Verification items for this drawing (mm, ordinates from the low corner). Round coordinates to 2 decimals unless told otherwise and drop trailing zeros. Loops run counter-clockwise (first coordinate to the right, second up) from the corner with the lowest first, then second, coordinate; pieces in that order, holes last. Notation, with made-up numbers: (43.5, -21) - (66.5, -21) arc R34 ccw to (66.5, 15) - close; hole circle Ø8 at (-16.5, -39). An arc over 180 degrees is marked (long way). Put each result on its own line as item: value. Start each with the question number.
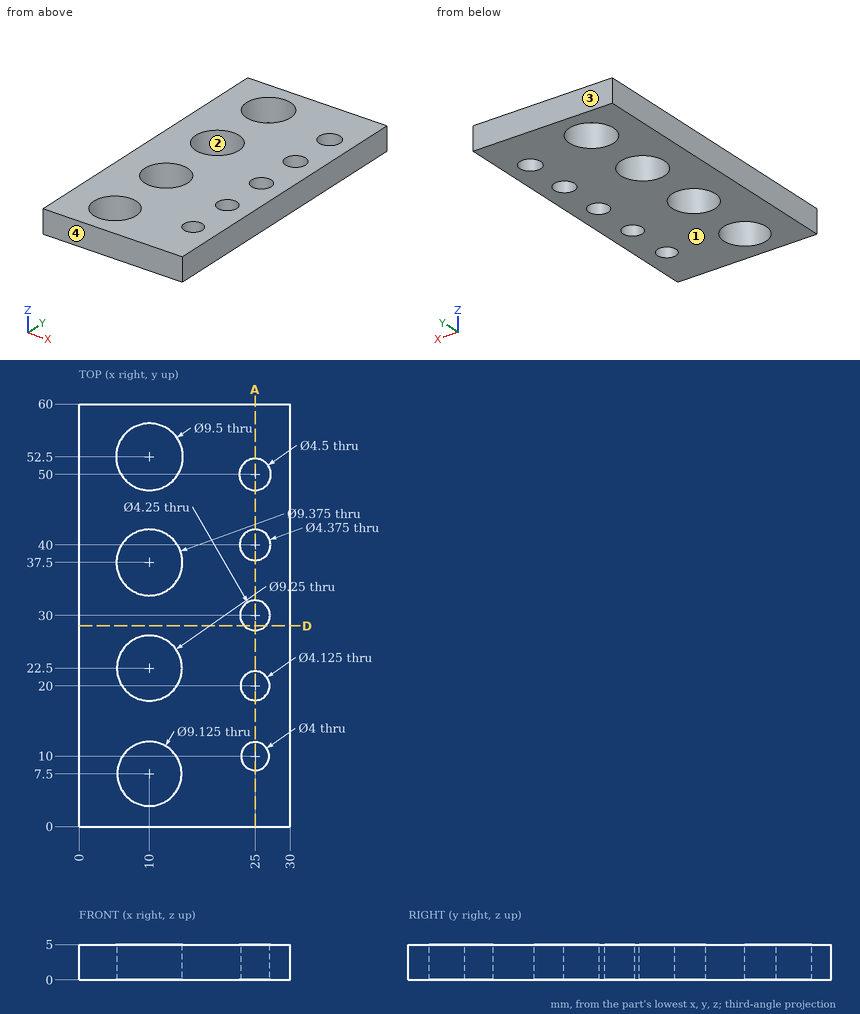
Q1. Draft check along Y on the marked faces 1, 2, 3 and 4. Enter one of: +Y half, -Y half, draft (parallel to the pull), parting line (faces both ways), or undercut.
Q2. Cross-section at D-D on y = 28.5. Enter the section's corners in (x, z), and give its area (3 significant figures).
Q3. Material ranges on line 1 (Y direction, x = 8, z = 1.8); line 2 (Y direction, x = 8.75, z = 1.35); line 3 (X direction, y = 28.5, z = 3.8), recorded low to high. Write a range as from..to.
Q4. Cross-section at A-A on x = 25. State how many separate pieces and enclosed holes the cut face has, and give its area (3 significant figures).
Answer list:
1. face 1: draft
1. face 2: undercut
1. face 3: +Y half
1. face 4: -Y half
2. outline: (0, 0) - (23.49, 0) - (23.49, 5) - (0, 5) - close; (26.51, 0) - (30, 0) - (30, 5) - (26.51, 5) - close
2. area: 135 mm2
3. line 1: y = 0..3.4, 11.6..18.33, 26.67..33.26, 41.74..48.19, 56.81..60
3. line 2: y = 0..3.11, 11.89..18.05, 26.95..32.98, 42.02..47.92, 57.08..60
3. line 3: x = 0..23.49, 26.51..30
4. separate pieces: 6
4. enclosed holes: 0
4. area: 194 mm2
